Could you check a few things on this model? Use its own coordinates, in mm. Face numbers are marked on the shaded views. A direction names the side the tool comes from. Coordinates: 2 decimals unless noted, no trailing zeros. Write each loop counter-clockwise with the first axis right and the second up, starting at its lowest first coordinate (ties: lowest second). Pieces come first, ordered by that corner, then holes.
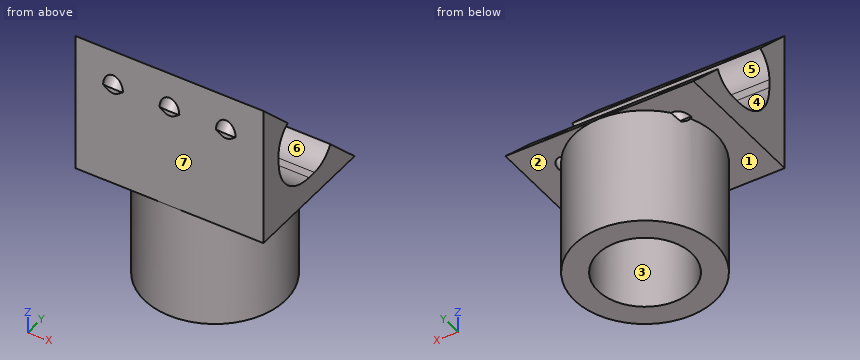
```python
from build123d import *

# Parameters (mm, degrees)
SKETCH1_R                            = 15
SKETCH1_R_2                          = 10
BOSS_EXTRUDE1_DEPTH                  = 25
SKETCH2_W                            = 40
SKETCH2_H                            = 30
BOSS_EXTRUDE2_DEPTH                  = 30
SKETCH3_R                            = 10
CUT_EXTRUDE1_DEPTH                   = 70.641941386
CUT_EXTRUDE2_DEPTH                   = 70.641941386
CUT_EXTRUDE6_DEPTH                   = 70.641941386
BOSS_EXTRUDE3_DEPTH                  = 40
FILLET1_R                            = 6
F_4_2_4_2_DIAMETER_HOLE1_D           = 4.2
F_4_2_4_2_DIAMETER_HOLE1_DEPTH       = 6
F_4_2_4_2_DIAMETER_HOLE1_CSINK_D     = 4.25
F_4_2_4_2_DIAMETER_HOLE1_CSINK_ANGLE = 90
F_4_2_4_2_DIAMETER_HOLE1_TIP         = 1.2618073


with BuildPart() as part:
    # Sketch1 → Boss-Extrude1 (new body)
    with BuildSketch(Plane.XY):
        Circle(SKETCH1_R)
        Circle(SKETCH1_R_2, mode=Mode.SUBTRACT)
    extrude(amount=BOSS_EXTRUDE1_DEPTH)

    # Sketch2 → Boss-Extrude2 (add)
    with BuildSketch(Plane.XY.offset(25)):
        Rectangle(SKETCH2_W, SKETCH2_H)
    extrude(amount=BOSS_EXTRUDE2_DEPTH)

    # Sketch3 → Cut-Extrude1 (cut, through all)
    with BuildSketch(Plane.ZY.offset(20)):
        with Locations(Location((40, 0, 0), (0, 0, 270))):
            Circle(SKETCH3_R)
    extrude(amount=-CUT_EXTRUDE1_DEPTH, mode=Mode.SUBTRACT)

    # Sketch4 → Cut-Extrude2 (cut, through all)
    with BuildSketch(Plane(origin=(20, 0, 0), x_dir=(0, 0, -1), z_dir=(1, 0, 0))):
        with BuildLine():
            Line((-30, 0), (-30, 15))
            Line((-30, 15), (-55, 15))
            Line((-55, 15), (-55, -10))
            Line((-55, -10), (-40, -10))
            ThreePointArc((-40, -10), (-32.928932188, -7.071067812), (-30, 0))
        make_face()
    extrude(amount=-CUT_EXTRUDE2_DEPTH, mode=Mode.SUBTRACT)

    # Sketch6 → Cut-Extrude6 (cut, through all)
    with BuildSketch(Plane(origin=(20, 0, 0), x_dir=(0, 0, -1), z_dir=(1, 0, 0))):
        Polygon((-25, 15), (-30, 10), (-30, 15), align=None)
        Polygon((-55, -10), (-55, -15), (-50, -10), align=None)
    extrude(amount=-CUT_EXTRUDE6_DEPTH, mode=Mode.SUBTRACT)

    # Sketch7 → Boss-Extrude3 (add)
    with BuildSketch(Plane.ZY.offset(20)):
        Polygon((30, 10), (33, 7), (30, 7), align=None)
        Polygon((50, -10), (47, -7), (47, -10), align=None)
    extrude(amount=-BOSS_EXTRUDE3_DEPTH)

    # Fillet1
    # the kernel refuses this fillet: 6 mm, written as the material it adds along each edge
    with BuildSketch(Plane(origin=(-20, -10, 47), x_dir=(0, 1, 0), z_dir=(1, 0, 0))) as fillet1_piece_1_section:
        with BuildLine():
            CenterArc((6, -5.196152423), FILLET1_R, 120, 60)
            Line((0, -5.196152423), (-0.12, -5.196152423))
            Line((-0.12, -5.196152423), (-0.12, 0))
            Line((-0.12, 0), (0, 0.12))
            ThreePointArc((0, 0.12), (1.5, 0.12), (2.94, 0.103923048))
            Line((2.94, 0.103923048), (3, 0))
        make_face()
    fillet1_piece_1 = extrude(amount=40, mode=Mode.PRIVATE)
    fillet1_piece_1 = split(fillet1_piece_1, bisect_by=Plane(origin=(0, -7.462685522, 47.462685522), z_dir=(0, -0.7071067811865475, -0.7071067811865477)), keep=Keep.TOP, mode=Mode.PRIVATE)
    add(fillet1_piece_1)
    with BuildSketch(Plane(origin=(-20, 7, 30), x_dir=(0, -1, 0), z_dir=(1, 0, 0))) as fillet1_piece_2_section:
        with BuildLine():
            CenterArc((5.196152423, -6), FILLET1_R, 90, 60)
            Line((0, -3), (-0.103923048, -2.94))
            ThreePointArc((-0.103923048, -2.94), (-0.12, -1.5), (-0.12, 0))
            Line((-0.12, 0), (0, 0.12))
            Line((0, 0.12), (5.196152423, 0.12))
            Line((5.196152423, 0.12), (5.196152423, 0))
        make_face()
    fillet1_piece_2 = extrude(amount=40, mode=Mode.PRIVATE)
    fillet1_piece_2 = split(fillet1_piece_2, bisect_by=Plane(origin=(0, 7.462685522, 32.537314478), z_dir=(0, -0.7071067811865477, -0.7071067811865475)), keep=Keep.TOP, mode=Mode.PRIVATE)
    add(fillet1_piece_2)

    # Ø4.2 (4.2) Diameter Hole1
    with Locations(Plane(origin=(0, 20, 20), x_dir=(1, 0, 0), z_dir=(0, 0.7071067811865475, 0.7071067811865477))):
        with Locations((12, -43.497474683), (0, -43.497474683), (-12, -43.497474683), (-12, -13.071067812), (0, -13.071067812), (12, -13.071067812)):
            CounterSinkHole(F_4_2_4_2_DIAMETER_HOLE1_D / 2, F_4_2_4_2_DIAMETER_HOLE1_CSINK_D / 2, depth=F_4_2_4_2_DIAMETER_HOLE1_DEPTH, counter_sink_angle=F_4_2_4_2_DIAMETER_HOLE1_CSINK_ANGLE)
            with Locations((0, 0, -(F_4_2_4_2_DIAMETER_HOLE1_DEPTH + F_4_2_4_2_DIAMETER_HOLE1_TIP / 2))):  # 118° drill point
                Cone(0, F_4_2_4_2_DIAMETER_HOLE1_D / 2, F_4_2_4_2_DIAMETER_HOLE1_TIP, mode=Mode.SUBTRACT)


solid = part.part
```
Item 1: Will these pins go through, and if not, where does the flat tip stop? pin 1 Ø4 at (y, z) = (5.5, 15.5) entering from +X; pin 2 Ø2 at (x, z) = (1, 40.5) entering from +Y; pin 3 Ø0.5 at (x, y) = (-8, 1) entering from +Z.
Item 2: I want a section at B-B, the plane z = 6. List the corners of the cut face in (x, y) for me, then the cut area to 3 significant figures.
Item 3: If we mould it in two halves opening along Y, with no side actions, what happens to the marked faces 5, 6 and 7? For each: released by +Y, released by -Y, zero draft, split by the parting line, or undercut.
Item 4: Which directions (+Z, -Z, +X, -X, +Y, -Y) give clear straight access to the entire face, cutting with the end or side of a thin tool? Please do the marked faces 1, 2, 3 and 4.
Item 5: I want a section at D-D, the plane x = 1. Count the separate pieces of the cut face and the enclosed holes in it, then the cut area to 3 significant figures.
Item 6: I want a section at C-C, the plane y = -1. List the corners of the cut face in (x, z) for me.
Item 7: I want a section at A-A, the plane x = -3. List the corners of the cut face in (y, z) for me.
Item 8: If I drill on line 1 along Y through (x, z) = (0, 18.5); line 2 along Z through (x, y) = (-12, 13.5); line 3 along Z through (x, y) = (-13, 6.5), over which ranges is the centre line in solid material (lowest first)?
Taken from the geometry:
1. pin 1: stops at x = 14.59
1. pin 2: stops at y = -9.99
1. pin 3: stops at z = 30
2. outline: circle Ø30 at (0, 0); hole circle Ø20 at (0, 0)
2. area: 393 mm2
3. face 5: released by +Y
3. face 6: undercut
3. face 7: released by -Y
4. face 1: -Z, -X
4. face 2: -Z, +X
4. face 3: -Z
4. face 4: +X, -X
5. separate pieces: 3
5. enclosed holes: 0
5. area: 498 mm2
6. outline: (-20, 25) - (-14.97, 25) - (-14.97, 0) - (-9.95, 0) - (-9.95, 25) - (9.95, 25) - (9.95, 0) - (14.97, 0) - (14.97, 25) - (20, 25) - (20, 30.05) - (-20, 30.05) - close
7. outline: (-15, 25) - (-14.7, 25) - (-14.7, 0) - (-9.54, 0) - (-9.54, 25) - (9.54, 25) - (9.54, 0) - (14.7, 0) - (14.7, 25) - (15, 25) - (7, 33) arc R6 cw to (1.8, 30) - (0, 30) arc R10 cw to (-10, 40) - (-10, 41.8) arc R6 cw to (-7, 47) - (-15, 55) - close
8. line 1: y = -15 to -10, 10 to 15
8. line 2: z = 25 to 26.5
8. line 3: z = 0 to 24.2, 27.6 to 32.27
